Design review of the part built by this model. Coordinates are the model's own, in mm. A direction names the side the tool comes from. Give positions to 0.01 mm unless a question says otherwise; leave off trailing zeros. Loops run counter-clockwise (first coordinate to the right, second up) from the corner with the lowest first, then second, coordinate; pieces in that order, holes last. Notation, with made-up numbers: M 59,40 L 103,40 A26 cw 103,71 Z; hole C -26,-1.75 d8. An arc over 180 degrees is marked long. Use a Markdown table: item, result. Add a question column.
(1) Draft analysis for pull direction X (two halves, no side actions). For faces 3 (the face through (63, 0, 25)), 4 (the face through (0, 9, 25)), 5 (the face through (47, 9.525, 29)), state which applies: pulls with the +X half, pulls with the -X half, needs draft (parallel to the pull), parting line crosses it, or undercut.
(2) For faces 1 (the face through (42.87, 14.35, 25.05)), 2 (the face through (63, 10, 50.8)), list the 3-axis set-ups (+Z, -Z, +X, -X, +Y, -Y) from which the entire face can be reached by the end or side of a thin tool; tool diameter is ignored.
(3) For probe 1 along X at (y, z) = (8.5, 25.4) (3 decimals); probe 2 along X at (y, z) = (10.5, 21); probe 3 along Z at (x, y) = (50.8, 13.25), list the stretches that pass through material, from the lowest coordinate up.
(4) Add section A-A, the plane x = 101.6. Give the boundary of the cut face in (y, z) (3 decimals).
(5) Add section D-D, the plane x = 25.4. Give the boundary of the cut face in (y, z), then the cut area to 3 significant figures.
(6) Add section B-B, the plane y = 7. Give the boundary of the cut face in (x, z) (3 decimals), then the cut area to 3 significant figures.
(7) Add section C-C, the plane z = 25.4. State how many separate pieces and enclosed holes the cut face has, then the cut area to 3 significant figures.
(8) Insertion check: pin 1 Ø14.5 at (x, z) = (50.8, 25.4) entering from +Y (3 decimals). The pin has a flat end and moves straight along its axis. Give the tip position at first contact, or say it passes through.
```python
from build123d import *

# Parameters (mm, degrees)
SKETCH1_W                                        = 127
SKETCH1_H                                        = 19.05
BOSS_EXTRUDE1_DEPTH                              = 50.8
F_1_2_CLEARANCE_HOLE1_D                          = 13.49248
CBORE_FOR_3_8_SOCKET_HEAD_CAP_SCREW1_D           = 9.8044
CBORE_FOR_3_8_SOCKET_HEAD_CAP_SCREW1_CBORE_D     = 15.875
CBORE_FOR_3_8_SOCKET_HEAD_CAP_SCREW1_CBORE_DEPTH = 9.525
CSK_FOR_12_FLAT_HEAD_MACHINE_SCREW1_D            = 5.7912
CSK_FOR_12_FLAT_HEAD_MACHINE_SCREW1_CSINK_D      = 11.1252
CSK_FOR_12_FLAT_HEAD_MACHINE_SCREW1_CSINK_ANGLE  = 82
F_1_4_0_2500_DOWEL_HOLE1_D                       = 6.35


with BuildPart() as part:
    # Sketch1 → Boss-Extrude1 (new body)
    with BuildSketch(Plane.XY):
        with Locations((63.5, 9.525)):
            Rectangle(SKETCH1_W, SKETCH1_H)
    extrude(amount=BOSS_EXTRUDE1_DEPTH)

    # 1/2 Clearance Hole1 (through all)
    with Locations(Plane(origin=(0, 19.05, 0), x_dir=(1, 0, 0), z_dir=(0, 1, 0))):
        with Locations((25.4, -25.4)):
            Hole(F_1_2_CLEARANCE_HOLE1_D / 2)

    # CBORE for 3/8 Socket Head Cap Screw1 (through all)
    with Locations(Plane(origin=(0, 19.05, 0), x_dir=(1, 0, 0), z_dir=(0, 1, 0))):
        with Locations((50.8, -25.4)):
            CounterBoreHole(CBORE_FOR_3_8_SOCKET_HEAD_CAP_SCREW1_D / 2, CBORE_FOR_3_8_SOCKET_HEAD_CAP_SCREW1_CBORE_D / 2, CBORE_FOR_3_8_SOCKET_HEAD_CAP_SCREW1_CBORE_DEPTH)

    # CSK for #12 Flat Head Machine Screw1 (through all)
    with Locations(Plane(origin=(0, 19.05, 0), x_dir=(1, 0, 0), z_dir=(0, 1, 0))):
        with Locations((76.2, -25.4)):
            CounterSinkHole(CSK_FOR_12_FLAT_HEAD_MACHINE_SCREW1_D / 2, CSK_FOR_12_FLAT_HEAD_MACHINE_SCREW1_CSINK_D / 2, counter_sink_angle=CSK_FOR_12_FLAT_HEAD_MACHINE_SCREW1_CSINK_ANGLE)

    # 1/4 (0.2500) Dowel Hole1 (through all)
    with Locations(Plane(origin=(0, 19.05, 0), x_dir=(1, 0, 0), z_dir=(0, 1, 0))):
        with Locations((101.6, -25.4)):
            Hole(F_1_4_0_2500_DOWEL_HOLE1_D / 2)


solid = part.part
```
Established:
| question | item | result |
|---|---|---|
| 1 | face 3 | needs draft |
| 1 | face 4 | pulls with the -X half |
| 1 | face 5 | undercut |
| 2 | face 1 | +Y |
| 2 | face 2 | +Z, +X, -X, +Y, -Y |
| 3 | probe 1 | 0 to 18.654, 32.146 to 45.898, 55.702 to 73.304, 79.096 to 98.425, 104.775 to 127 |
| 3 | probe 2 | 0 to 20.29, 30.51 to 44.19, 57.41 to 127 |
| 3 | probe 3 | 0 to 17.46, 33.34 to 50.8 |
| 4 | outline | M 0,0 L 19.05,0 L 19.05,22.225 L 0,22.225 Z; M 0,28.575 L 19.05,28.575 L 19.05,50.8 L 0,50.8 Z |
| 5 | outline | M 0,0 L 19.05,0 L 19.05,18.65 L 0,18.65 Z; M 0,32.15 L 19.05,32.15 L 19.05,50.8 L 0,50.8 Z |
| 5 | area | 711 mm^2 |
| 6 | outline | M 0,0 L 127,0 L 127,50.8 L 0,50.8 Z; hole C 25.4,25.4 d13.492; hole C 50.8,25.4 d9.804; hole C 76.2,25.4 d5.791; hole C 101.6,25.4 d6.35 |
| 6 | area | 6,180 mm^2 |
| 7 | separate pieces | 5 |
| 7 | enclosed holes | 0 |
| 7 | area | 1,680 mm^2 |
| 8 | pin 1 | y = 9.525 |
